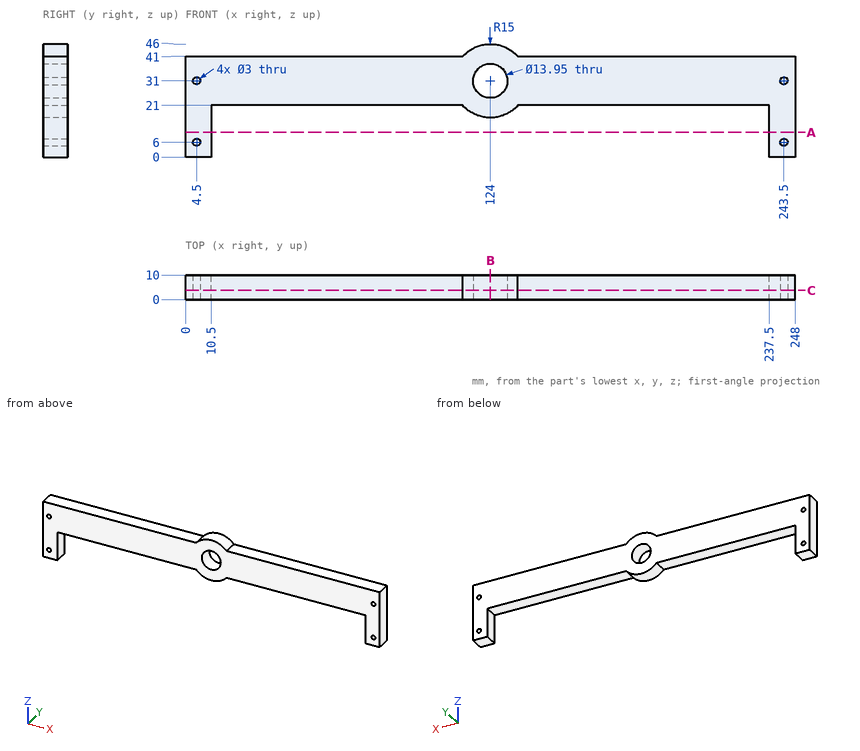
Can you work these out from the drawing? Everything is in mm from the part's minimum corner. Round coordinates to 2 decimals unless told otherwise and drop trailing zeros. Order: outer loops, then holes, each group sorted by start corner. A loop starts at its lowest first (then second) coordinate and runs counter-clockwise, first axis right, second up. Notation, with made-up numbers: M 57,-19.75 L 61,-19.75 A19 cw 61,-0.75 Z; hole C -17.5,25.25 d11. An arc over 180 degrees is marked long. Answer as CSV lines item,"result".
Item 1: For pin 1 (3 mm diameter, centred on x = 182, y = 3, fed in from +Z); pin 2 (5 mm diameter, centred on x = 26.5, y = 6, fed in from -Z), each with a flat end and sliding along its axis, tell me the tip position at first contact or that it passes through.
From the geometry:
pin 1,"z = 41"
pin 2,"z = 21"
Item 2: Imagine slicing it at B-B on x = 124. List the corners of the cut face in (y, z) for me (3 decimals).
From the geometry:
outline,"M 0,16 L 10,16 L 10,24.025 L 0,24.025 Z; M 0,37.975 L 10,37.975 L 10,46 L 0,46 Z"
Item 3: Imagine slicing it at C-C on y = 3.75. List the corners of the cut face in (x, z) for me (3 decimals), and give its area (3 significant figures).
From the geometry:
outline,"M 0,0 L 10.5,0 L 10.5,21 L 112.82,21 A15 ccw 135.18,21 L 237.5,21 L 237.5,0 L 248,0 L 248,41 L 135.18,41 A15 ccw 112.82,41 L 0,41 Z; hole C 4.5,6 d3; hole C 4.5,31 d3; hole C 124,31 d13.95; hole C 243.5,6 d3; hole C 243.5,31 d3"
area,"5,370 mm2"
Item 4: Imagine slicing it at A-A on z = 10. List the corners of the cut face in (x, y) for me, and give its area (3 significant figures).
From the geometry:
outline,"M 0,0 L 10.5,0 L 10.5,10 L 0,10 Z; M 237.5,0 L 248,0 L 248,10 L 237.5,10 Z"
area,"210 mm2"
Item 5: Please list where these lines run through material, in increasing order: L1, parallel to Z at x = 243.5, y = 2.5; L2, parallel to X at y = 2.25, z = 6; L3, parallel to X at y = 2.5, z = 31 (3 decimals). Write a range as [from, to].
From the geometry:
L1,"[0, 4.5], [7.5, 29.5], [32.5, 41]"
L2,"[0, 3], [6, 10.5], [237.5, 242], [245, 248]"
L3,"[0, 3], [6, 117.025], [130.975, 242], [245, 248]"
